Verification items for the finished model (mm, model axes). A direction names the side the tool comes from. Give positions to 0.01 mm unless a question says otherwise; leave off trailing zeros. Loops run counter-clockwise (first coordinate to the right, second up) from the corner with the lowest first, then second, coordinate; pieces in that order, holes last. Notation, with made-up numbers: (-9.5, -34) - (9.5, -34) arc R22 cw to (9.5, -13) - close; hole circle Ø10 at (-12.75, 17). An arc over 180 degrees is marked (long way). Answer in a Markdown table with one row per item.
```python
from build123d import *

# Parameters (mm, degrees)
ESBO_O1_W                = 90
ESBO_O1_H                = 93
RESSALTO_EXTRUS_O1_DEPTH = 9.53
ESBO_O3_R                = 32.51
CORTE_EXTRUS_O2_DEPTH    = 66.406963697
ESBO_O2_R                = 2
CORTE_EXTRUS_O1_DEPTH    = 19
CORTE_EXTRUS_O4_REACH    = 67.407
ESBO_O5_W                = 27.5
ESBO_O5_H                = 13
CORTE_EXTRUS_O5_REACH    = 67.407
ESBO_O6_W                = 7
ESBO_O6_H                = 26.329700269
CORTE_EXTRUS_O6_REACH    = 80.481
ESBO_O7_R                = 2.5
CORTE_EXTRUS_O8_DEPTH    = 66.406963697


with BuildPart() as part:
    # Esboço1 → Ressalto-extrusão1 (new body)
    with BuildSketch(Plane(origin=(0, 0, 0), x_dir=(1, 0, 0), z_dir=(0, 1, 0))):
        Rectangle(ESBO_O1_W, ESBO_O1_H)
    extrude(amount=RESSALTO_EXTRUS_O1_DEPTH)

    # Esboço3 → Corte-extrusão2 (cut, through all)
    with BuildSketch(Plane(origin=(0, 9.53, 0), x_dir=(1, 0, 0), z_dir=(0, 1, 0))):
        with Locations(Location((0, 3.5, 0), (0, 0, 270))):
            Circle(ESBO_O3_R)
    extrude(amount=-CORTE_EXTRUS_O2_DEPTH, mode=Mode.SUBTRACT)

    # Esboço2 → Corte-extrusão1 (cut)
    with BuildSketch(Plane(origin=(0, 0, -46.5), x_dir=(-1, 0, 0), z_dir=(0, 0, -1))):
        with Locations((-40, 4.765)):
            Circle(ESBO_O2_R)
        with Locations((-25, 4.765)):
            Circle(ESBO_O2_R)
        with Locations((25, 4.765)):
            Circle(ESBO_O2_R)
        with Locations((40, 4.765)):
            Circle(ESBO_O2_R)
    extrude(amount=-CORTE_EXTRUS_O1_DEPTH, mode=Mode.SUBTRACT)

    # Esboço5 → Corte-extrusão4 (cut, up to next)
    with BuildSketch(Plane(origin=(0, 9.53, 0), x_dir=(1, 0, 0), z_dir=(0, 1, 0)), mode=Mode.PRIVATE) as corte_extrus_o4_sk1:
        with Locations((31.25, -40)):
            Rectangle(ESBO_O5_W, ESBO_O5_H)
    corte_extrus_o4_tool1 = extrude(corte_extrus_o4_sk1.sketch, amount=-CORTE_EXTRUS_O4_REACH, mode=Mode.PRIVATE) & part.part
    # Esboço5 → Corte-extrusão4 (cut, up to next)
    with BuildSketch(Plane(origin=(0, 9.53, 0), x_dir=(1, 0, 0), z_dir=(0, 1, 0)), mode=Mode.PRIVATE) as corte_extrus_o4_sk2:
        with Locations((-31.25, -40)):
            Rectangle(ESBO_O5_W, ESBO_O5_H)
    corte_extrus_o4_tool2 = extrude(corte_extrus_o4_sk2.sketch, amount=-CORTE_EXTRUS_O4_REACH, mode=Mode.PRIVATE) & part.part
    add(corte_extrus_o4_tool1.solids().sort_by_distance((31.25, 9.53, 40))[0], mode=Mode.SUBTRACT)
    add(corte_extrus_o4_tool2.solids().sort_by_distance((-31.25, 9.53, 40))[0], mode=Mode.SUBTRACT)

    # Esboço6 → Corte-extrusão5 (cut, up to next)
    with BuildSketch(Plane(origin=(0, 9.53, 0), x_dir=(1, 0, 0), z_dir=(0, 1, 0)), mode=Mode.PRIVATE) as corte_extrus_o5_sk1:
        with Locations((0, -33.335149866)):
            Rectangle(ESBO_O6_W, ESBO_O6_H)
    corte_extrus_o5_tool1 = extrude(corte_extrus_o5_sk1.sketch, amount=-CORTE_EXTRUS_O5_REACH, mode=Mode.PRIVATE) & part.part
    add(corte_extrus_o5_tool1.solids().sort_by_distance((0, 9.53, 33.33515))[0], mode=Mode.SUBTRACT)

    # Corte-extrusão6: up to this face of the body (flat: up to its plane)
    corte_extrus_o6_end = Plane(part.part.faces().sort_by_distance((17.5, 4.765, 40))[0])
    # Esboço7 → Corte-extrusão6 (cut, up to the picked face)
    with BuildSketch(Plane.ZY.offset(17.5), mode=Mode.PRIVATE) as corte_extrus_o6_sk1:
        with Locations((41.5, 4.765)):
            Circle(ESBO_O7_R)
    corte_extrus_o6_tool1 = split(extrude(corte_extrus_o6_sk1.sketch, amount=-CORTE_EXTRUS_O6_REACH, mode=Mode.PRIVATE), bisect_by=corte_extrus_o6_end, keep=Keep.BOTH, mode=Mode.PRIVATE)
    add(corte_extrus_o6_tool1.solids().sort_by(Axis((-17.5, 4.765, 41.5), (1, 0, 0)))[0], mode=Mode.SUBTRACT)

    # Esboço9 → Corte-extrusão8 (cut, through all)
    with BuildSketch(Plane(origin=(0, 9.53, 0), x_dir=(-1, 0, 0), z_dir=(0, 1, 0))):
        Polygon((45, 28.5), (25.5, 28.5), (17.5, 33.5), (45, 33.5), align=None)
        Polygon((-25.5, 28.5), (-17.5, 33.5), (-45, 33.5), (-45, 28.5), align=None)
    extrude(amount=-CORTE_EXTRUS_O8_DEPTH, mode=Mode.SUBTRACT)


solid = part.part
```
Q1. Sectioned sample at C-C (x = 21). Record the cut outline in (y, z), and give its area (3 significant figures).
Completed:
| item | result |
|---|---|
| outline | (0, -46.5) - (9.53, -46.5) - (9.53, -28.32) - (0, -28.32) - close; (0, 21.32) - (9.53, 21.32) - (9.53, 31.31) - (0, 31.31) - close |
| area | 269 mm^2 |
Q2. Draft check along Z on faces 1 (the face through (40, 5, -27.5)), 2 (the face through (-10.6, 3.81, 43.81)), 3 (the face through (-17.5, 4.8, 38.6)). Enter one of: +Z half, -Z half, draft (parallel to the pull), parting line (faces both ways), or undercut.
Completed:
| item | result |
|---|---|
| face 1 | -Z half |
| face 2 | undercut |
| face 3 | draft |
Q3. Sectioned sample at B-B (x = 10.5). Record the cut outline in (y, z) (3 decimals).
Completed:
| item | result |
|---|---|
| outline | (0, -46.5) - (9.53, -46.5) - (9.53, -34.268) - (0, -34.268) - close; (0, 27.268) - (9.53, 27.268) - (9.53, 46.5) - (0, 46.5) - close; hole circle Ø5 at (4.765, 41.5) |
Q4. Tool access check on faces 4 (the face through (17.5, 4.8, 38.6)), 5 (the face through (-35, 5, 28.5)), 6 (the face through (-21, 0, -32)), 7 (the face through (-23.53, 6.12, -37.13)), 8 (the face through (3.5, 5, 38)). Record the directions out of +Z, -Z, +X, -X, +Y, -Y that give a thin tool (end or side, any length) a straight path to the whole face; none if there is none.
Completed:
| item | result |
|---|---|
| face 4 | +Z, +X, +Y, -Y |
| face 5 | +Z, -X, +Y, -Y |
| face 6 | +Z, -Z, +X, -X, -Y |
| face 7 | -Z |
| face 8 | +Z, +Y, -Y |
Q5. Thickness scan on line 1 (Y direction, x = -25, z = -41) (3 decimals); line 2 (Y direction, x = 14.25, z = 41.5) (3 decimals); line 3 (Z direction, x = -10, y = 6). Record the ranges inside material, lowest first.
Completed:
| item | result |
|---|---|
| line 1 | 0 to 2.765, 6.765 to 9.53 |
| line 2 | 0 to 2.265, 7.265 to 9.53 |
| line 3 | -46.5 to -34.43, 27.43 to 39.33, 43.67 to 46.5 |
Q6. Sectioned sample at A-A (z = 36). Record the cut outline in (x, y), and give its area (3 significant figures).
Completed:
| item | result |
|---|---|
| outline | (-17.5, 0) - (-3.5, 0) - (-3.5, 9.53) - (-17.5, 9.53) - close; (3.5, 0) - (17.5, 0) - (17.5, 9.53) - (3.5, 9.53) - close |
| area | 267 mm^2 |
Q7. Sectioned sample at D-D (x = -40). Record the cut outline in (y, z) (3 decimals).
Completed:
| item | result |
|---|---|
| outline | (0, -46.5) - (2.765, -46.5) - (2.765, -27.5) - (6.765, -27.5) - (6.765, -46.5) - (9.53, -46.5) - (9.53, 28.5) - (0, 28.5) - close |
Q8. Go/stop test with flat-tipped pins: P1, Ø2, axis at x = 25, y = 5, coming from the -Z side; P2, Ø5, axis at x = 40, y = 4.765, coming from the +Z side; P3, Ø1.5, axis at x = -2.5, y = 3.5, coming from the +Z side. Record where each tip stops, or that it passes through.
Completed:
| item | result |
|---|---|
| P1 | z = -27.5 |
| P2 | z = 28.5 |
| P3 | z = -35.85 |
